Can you work these out from the model? Positions are in its coordinate system, mm. A direction names the side the tool comes from. Give positions to 0.01 mm unless a question says otherwise; leave off trailing zeros. Order: outer loops, then holes, each group sorted by start corner. A loop starts at its lowest first (then second) coordinate and runs counter-clockwise, first axis right, second up.
Item 1: I want a section at A-A, the plane z = 0. Write out the boundary of the cut face in (x, y) (3 decimals), then the cut area to 3 significant figures.
Item 2: I want a section at B-B, the plane x = 0. Write out the boundary of the cut face in (y, z) (3 decimals).
Item 3: Which directions (+Z, -Z, +X, -X, +Y, -Y) give clear straight access to the entire face, cutting with the end or side of a thin tool? Please do faces 4 (the flat face through (0, -4.5, -13)), 5 (the flat face through (0, 10, 12.5)), 6 (the cylindrical face through (14.299, 10.218, -15.846)).
Item 4: I want a section at C-C, the plane y = -17. Write out the boundary of the cut face in (x, z) (3 decimals).
Item 5: I want a section at D-D, the plane y = -2.5. Write out the boundary of the cut face in (x, z) (3 decimals).
Item 6: I'm going to push flat-ended pins straight in: pin 1 Ø3 at (x, z) = (-1.5, -14) entering from +Y; pin 2 Ø6.5 at (x, y) = (1.5, -14.5) entering from +Z; pin 3 Ø3 at (y, z) = (-1.5, -14.5) entering from +X. Where does each tip first touch, or does it pass through?
Item 7: If we mould it in two halves opening along X, with no side actions, what happens to faces 1 (the cylindrical face through (2.17, -26.97, 9.76)), 2 (the flat face through (4.125, -11, 0)), 3 (the flat face through (-4.3, -29, -0.1))? For each: +X half, -X half, draft (parallel to the pull), parting line (faces both ways), or undercut.
Item 8: If I drill on line 1 along Z through (x, y) = (1, -10) (3 decimals); line 2 along X through (y, z) = (11.5, 8); line 3 along X through (y, z) = (-19.5, -1) (3 decimals), over which ranges is the centre line in solid material (lowest first)?
```python
from build123d import *

# Parameters (mm, degrees)
F0_W     = 10
F0_H     = 4
F0_W_2   = 22.5
F0_H_2   = 25
F2_W     = 8.25
F2_H     = 8.25
F3_DEPTH = 41.501
F2_W_2   = 13.25
F2_H_2   = 25
F4_DEPTH = 6
F2_W_3   = 6.375
F5_DEPTH = 4.5
F6_R     = 2
F8_W     = 6.5
F8_H     = 6.5
F9_DEPTH = 25


with BuildPart() as f1:
    # F0 (on Top) → F1 (revolve)
    with BuildSketch(Plane.XY):
        with Locations((-5, -27)):
            Rectangle(F0_W, F0_H)
        Polygon((0, -25), (0, -12.5), (-22.5, -12.5), (-10, -25), align=None)
        with Locations((-11.25, 0)):
            Rectangle(F0_W_2, F0_H_2)
    revolve(axis=Axis((0, -8.25, 0), (0, -1, 0)))

    # F2 (on face) → F3 (cut, through all)
    with BuildSketch(Plane(origin=(0, 12.5, 0), x_dir=(-1, 0, 0), z_dir=(0, 1, 0))):
        Rectangle(F2_W, F2_H)
    extrude(amount=-F3_DEPTH, mode=Mode.SUBTRACT)

    # F2 (on face) → F4 (cut)
    with BuildSketch(Plane(origin=(0, 12.5, 0), x_dir=(-1, 0, 0), z_dir=(0, 1, 0))):
        Rectangle(F2_W_2, F2_H_2)
        Rectangle(F2_W, F2_H, mode=Mode.SUBTRACT)
    extrude(amount=-F4_DEPTH, mode=Mode.SUBTRACT)

    # F2 (on face) → F5 (cut)
    with BuildSketch(Plane(origin=(0, 12.5, 0), x_dir=(-1, 0, 0), z_dir=(0, 1, 0))):
        with BuildLine():
            Line((13, -18.3643676722), (13, -12.5))
            Line((13, -12.5), (6.625, -12.5))
            Line((6.625, -12.5), (-6.625, -12.5))
            Line((-6.625, -12.5), (-13, -12.5))
            Line((-13, -12.5), (-13, -18.3643676722))
            ThreePointArc((-13, -18.3643676722), (-6.8209870025, -21.4411785197), (0, -22.5))
            ThreePointArc((0, -22.5), (6.8209870025, -21.4411785197), (13, -18.3643676722))
        make_face()
        with Locations((9.8125, 0)):
            Rectangle(F2_W_3, F2_H_2)
        Rectangle(F2_W_2, F2_H_2)
        Rectangle(F2_W, F2_H, mode=Mode.SUBTRACT)
        with Locations((-9.8125, 0)):
            Rectangle(F2_W_3, F2_H_2)
    extrude(amount=-F5_DEPTH, mode=Mode.SUBTRACT)

    # F6
    f6_edges = [f1.edges().sort_by_distance(p)[0] for p in [
        (13, 10.25, -18.364368),
        (-13, 10.25, -18.364368),
    ]]
    fillet(f6_edges, radius=F6_R)

    # F8 (on offset) → F9 (cut)
    with BuildSketch(Plane.XY.offset(-25)):
        with Locations((0, -1.25)):
            Rectangle(F8_W, F8_H)
    extrude(amount=F9_DEPTH, mode=Mode.SUBTRACT)


solid = f1.part
```
Results list:
1. outline: (-22.5, -12.5) - (-10, -25) - (-10, -29) - (-4.125, -29) - (-4.125, 6.5) - (-6.625, 6.5) - (-6.625, 8) - (-13, 8) - (-13, 12.5) - (-22.5, 12.5) - close; (4.125, -29) - (10, -29) - (10, -25) - (22.5, -12.5) - (22.5, 12.5) - (13, 12.5) - (13, 8) - (6.625, 8) - (6.625, 6.5) - (4.125, 6.5) - close
1. area: 1,180 mm2
2. outline: (-29, -10) - (-25, -10) - (-12.5, -22.5) - (-4.5, -22.5) - (-4.5, -4.125) - (-29, -4.125) - close; (-29, 4.125) - (6.5, 4.125) - (6.5, 12.5) - (12.5, 12.5) - (12.5, 22.5) - (-12.5, 22.5) - (-25, 10) - (-29, 10) - close; (2, -22.5) - (8, -22.5) - (8, -12.5) - (6.5, -12.5) - (6.5, -4.125) - (2, -4.125) - close
3. face 4: -Z
3. face 5: +Y
3. face 6: -Z, +Y
4. outline: circle Ø36 at (0, 0); hole (-4.125, -4.125) - (4.125, -4.125) - (4.125, 4.125) - (-4.125, 4.125) - close
5. outline: (-4.125, -4.125) - (-4.125, 4.125) - (4.125, 4.125) - (4.125, -4.125) - (3.25, -4.125) - (3.25, -22.264) arc R22.5 ccw (long way) to (-3.25, -22.264) - (-3.25, -4.125) - close
6. pin 1: stops at y = 8
6. pin 2: stops at z = 22.5
6. pin 3: stops at x = 18.36
7. face 1: parting line
7. face 2: undercut
7. face 3: draft
8. line 1: z = -22.478 to -4.125, 4.125 to 22.478
8. line 2: x = -21.03 to -13, 13 to 21.03
8. line 3: x = -15.468 to -4.125, 4.125 to 15.468
